```python
from build123d import *
from build123d.topology import SkipClean

# Parameters (mm, degrees)
BOSS_EXTRUDE1_DEPTH = 18
SKETCH1_3_R         = 7
BOSS_EXTRUDE2_DEPTH = 12
SKETCH2_R           = 12
SKETCH2_R_2         = 6
BOSS_EXTRUDE3_DEPTH = 9
RIB1_START          = -3
RIB1_DEPTH          = 6
CHAMFER1_SIZE       = 8
CHAMFER1_SIZE2      = 15
CHAMFER2_SIZE       = 15
CHAMFER2_SIZE2      = 8
SKETCH2_2_R         = 6
CUT_EXTRUDE1_DEPTH  = 72.505244563


# Read off the part's stored shape, not the designer's step: Rib1
with BuildPart() as part:
    # Sketch1 → Boss-Extrude1 (new, symmetric)
    with BuildSketch(Plane.XY):
        with BuildLine():
            Line((18, 0), (24, 0))
            ThreePointArc((24, 0), (0, 24), (-24, 0))
            Line((-24, 0), (-18, 0))
            ThreePointArc((-18, 0), (0, 18), (18, 0))
        make_face()
        with BuildLine():
            Line((55, 6), (23.237900077, 6))
            ThreePointArc((23.237900077, 6), (23.80871271, 3.02410302), (24, 0))
            Line((24, 0), (55, 0))
            Line((55, 0), (55, 6))
        make_face()
    extrude(amount=BOSS_EXTRUDE1_DEPTH, both=True)

    # Sketch1<3> → Boss-Extrude2 (add, symmetric)
    with BuildSketch(Plane.XY):
        with BuildLine():
            Line((-24, 36), (-24, 0))
            ThreePointArc((-24, 0), (-16.970562748, 16.970562748), (0, 24))
            Line((0, 24), (0, 36))
            ThreePointArc((0, 36), (-12, 48), (-24, 36))
        make_face()
        with Locations((-12, 36)):
            Circle(SKETCH1_3_R, mode=Mode.SUBTRACT)
    extrude(amount=BOSS_EXTRUDE2_DEPTH, both=True)

    # Sketch2 → Boss-Extrude3 (add)
    with BuildSketch(Plane(origin=(0, 6, 0), x_dir=(1, 0, 0), z_dir=(0, 1, 0))):
        with Locations((40, 0)):
            Circle(SKETCH2_R)
        with Locations(Location((40, 0, 0), (0, 0, 180))):
            Circle(SKETCH2_R_2, mode=Mode.SUBTRACT)
    extrude(amount=BOSS_EXTRUDE3_DEPTH)

    # Rib1 outline → Rib1 (add)
    with SkipClean():  # the faces are left unmerged after this step: merging them gives an invalid solid
        with BuildSketch(Plane.XY.offset(RIB1_START)):
            with BuildLine():
                Line((28.381049961, 14.714212529), (0, 36))
                Line((0, 36), (0, 24))
                ThreePointArc((0, 24), (14.696938456, 18.973665961), (23.237900077, 6))
                Line((23.237900077, 6), (30, 6))
                Line((30, 6), (30, 13.5))
                Line((30, 13.5), (28.381049961, 14.714212529))
            make_face()
        extrude(amount=RIB1_DEPTH)

    # Chamfer1
    chamfer1_edges = [part.edges().sort_by_distance(p)[0] for p in [
        (55, 3, 18),
    ]]
    chamfer1_side = [part.faces().sort_by_distance(p)[0] for p in [
        (55, 3, 0),
    ]]
    chamfer(chamfer1_edges, length=CHAMFER1_SIZE, length2=CHAMFER1_SIZE2, reference=chamfer1_side[0])

    # Chamfer2
    chamfer2_edges = [part.edges().sort_by_distance(p)[0] for p in [
        (55, 3, -18),
    ]]
    chamfer2_side = [part.faces().sort_by_distance(p)[0] for p in [
        (36.5, 0.825651258, -18),
    ]]
    chamfer(chamfer2_edges, length=CHAMFER2_SIZE, length2=CHAMFER2_SIZE2, reference=chamfer2_side[0])

    # Sketch2<2> → Cut-Extrude1 (cut, through all)
    with BuildSketch(Plane(origin=(0, 6, 0), x_dir=(1, 0, 0), z_dir=(0, 1, 0))):
        with Locations(Location((40, 0, 0), (0, 0, 180))):
            Circle(SKETCH2_2_R)
    extrude(amount=-CUT_EXTRUDE1_DEPTH, mode=Mode.SUBTRACT)


solid = part.part
```
For this review, take the finished solid that the model builds, in its own axes (mm). A direction names the side the tool comes from. Round coordinates to 2 decimals unless told otherwise and drop trailing zeros. Write each loop counter-clockwise with the first axis right and the second up, starting at its lowest first coordinate (ties: lowest second). Pieces come first, ordered by that corner, then holes. Notation, with made-up numbers: M -5,56.25 L 49,56.25 A15 ccw 49,84.25 Z; hole C -7.75,46 d9. An arc over 180 degrees is marked long. One line per item, written item: value. Start each with the question number.
(1) We need section D-D (y = 21). Give the boundary of the cut face in (x, z), and give its area (3 significant figures).
(2) Machinability: for faces 4 (the flat face through (-18, 30, 12)), 5 (the flat face through (0, 30, 8)), 6 (the flat face through (0, 30, -7)), 7 (the flat face through (15, 21, 3)), which of the approach directions +Z, -Z, +X, -X, +Y, -Y give a long, thin tool a straight path to every point of the face, cutting with its end or side? Answer none if there is none.
(3) The part is to be moulded in two halves that separate along Y. For faces 1 (the flat face through (15, 21, -3)), 2 (the cylindrical face through (-12.91, 42.94, -0.17)), 3 (the cylindrical face through (0, 18, 0)), say which applies: released by +Y, released by -Y, zero draft, split by the parting line, or undercut.
(4) Wall thickness on line 1 (Z direction, x = 40, y = 2); line 2 (X direction, y = 11, z = 10); line 3 (Z direction, x = -12.5, y = 25.5): over which ranges is each line inside the solid? List them lowest first.
(5) We need section A-A (y = 3.5). Give the boundary of the cut face in (x, z).
(6) We need section B-B (z = -11). Give the boundary of the cut face in (x, y) (3 decimals), and give its area (3 significant figures).
(7) We need section C-C (x = 39). Give the boundary of the cut face in (y, z).
(8) Insertion check: pin 1 (12 mm diameter, centred on x = -13, y = 28.5, fed in from +Z); pin 2 (8 mm diameter, centred on y = 33.5, z = 1, fed in from +X); pin 3 (12.5 mm diameter, centred on x = -12, y = 36, fed in from +Z); pin 4 (8 mm diameter, centred on y = 19.5, z = 10, fed in from +X). Each pin has a flat end and moves straight along its axis. Give the tip position at first contact, or say it passes through.
Result:
1. outline: M -24,-12 L -11.62,-12 L -11.62,-18 L 11.62,-18 L 11.62,-3 L 20,-3 L 20,3 L 11.62,3 L 11.62,18 L -11.62,18 L -11.62,12 L -24,12 Z
1. area: 1,180 mm²
2. face 4: +Z, -X, +Y
2. face 5: +Z, +X, +Y
2. face 6: -Z, +X, +Y
2. face 7: +Z, +Y
3. face 1: zero draft
3. face 2: undercut
3. face 3: released by -Y
4. line 1: -18 to -6, 6 to 18
4. line 2: -24 to -14.25, 14.25 to 21.33, 33.37 to 46.63
4. line 3: -12 to 12
5. outline: M -24,-12 L -23.74,-12 L -23.74,-18 L -17.66,-18 L -17.66,18 L -23.74,18 L -23.74,12 L -24,12 Z; M 17.66,-18 L 40,-18 L 55,-10 L 55,10 L 40,18 L 17.66,18 Z; hole C 40,0 d12
6. outline: M -24,0 L -18,0 A18 cw 18,0 L 53.125,0 L 53.125,6 L 44.796,6 L 44.796,15 L 35.204,15 L 35.204,6 L 23.238,6 A24 ccw 0,24 L 0,36 A12 ccw -24,36 Z; hole C -12,36 d14
6. area: 1,140 mm²
7. outline: M 0,-18 L 6,-18 L 6,-11.96 L 15,-11.96 L 15,-5.92 L 0,-5.92 Z; M 0,5.92 L 15,5.92 L 15,11.96 L 6,11.96 L 6,18 L 0,18 Z
8. pin 1: z = 12
8. pin 2: x = 8.67
8. pin 3: through
8. pin 4: x = 18.32
